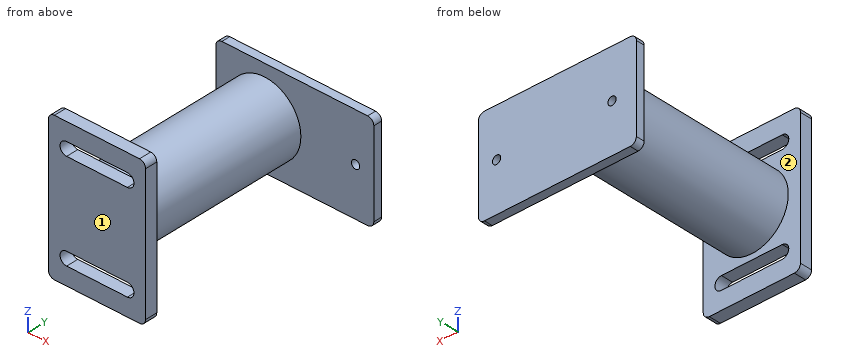
Autodesk Inventor part; units mm, degrees
ref_plane "YZ Plane" through (0, 0, 0) normal (1, 0, 0) x (0, 1, 0)
ref_plane "XZ Plane" through (0, 0, 0) normal (0, 1, 0) x (-1, 0, 0)
ref_plane "XY Plane" through (0, 0, 0) normal (0, 0, 1) x (1, 0, 0)
sketch "Sketch2" plane through (0, 0, 0) normal (0, 1, 0) x (-1, 0, 0)
  line L0 (-25.4, 38.1) -> (25.4, 38.1)
  line L1 (25.4, 38.1) -> (25.4, -38.1)
  line L2 (25.4, -38.1) -> (-25.4, -38.1)
  line L3 (-25.4, -38.1) -> (-25.4, 38.1)
  point P0 (0, 0)
  dimension "d0" = 50.8
  dimension "d1" = 76.2
  dimension "d2" = 25.4
  dimension "d3" = 38.1
extrude "Extrusion1" add sketch "Sketch2" against normal blind 6.35
sketch "Sketch3" plane through (0, 0, 0) normal (0, 1, 0) x (1, 0, 0)
  circle A0 centre (0, 0) radius 19.05
  dimension "d6" = 38.1
extrude "Extrusion2" add sketch "Sketch3" along normal blind 88.9
sketch "Sketch4" plane through (0, 0, 0) normal (0, 1, 0) x (1, 0, 0)
  circle A0 centre (0, 0) radius 19.05
  line L0 (-15.875, 28.829) -> (15.875, 28.829)
  line L1 (15.875, 28.829) -> (15.875, 21.971)
  line L2 (15.875, 21.971) -> (-15.875, 21.971)
  line L3 (-15.875, 21.971) -> (-15.875, 28.829)
  line L4 (-15.875, -21.971) -> (15.875, -21.971)
  line L5 (15.875, -21.971) -> (15.875, -28.829)
  line L6 (15.875, -28.829) -> (-15.875, -28.829)
  line L7 (-15.875, -28.829) -> (-15.875, -21.971)
  line L8 (-15.875, 25.4) -> (15.875, 25.4)
  line L9 (-15.875, -25.4) -> (15.875, -25.4)
  circle A1 centre (-15.875, 25.4) radius 3.429
  circle A2 centre (15.875, 25.4) radius 3.429
  circle A3 centre (15.875, -25.4) radius 3.429
  circle A4 centre (-15.875, -25.4) radius 3.429
  dimension "d10" = 6.858
  dimension "d11" = 6.858
  dimension "d12" = 25.4
  dimension "d14" = 25.4
  dimension "d15" = 31.75
  dimension "d16" = 31.75
  dimension "d17" = 15.875
  dimension "d18" = 15.875
sketch "Sketch5" plane through (0, 88.9, 0) normal (0, 1, 0) x (1, 0, 0)
  circle A0 centre (0, 0) radius 19.05
  line L0 (-25.4, 25.4) -> (57.15, 25.4)
  line L1 (57.15, 25.4) -> (57.15, -25.4)
  line L2 (57.15, -25.4) -> (-25.4, -25.4)
  line L3 (-25.4, -25.4) -> (-25.4, 25.4)
  dimension "d19" = 50.8
  dimension "d20" = 82.55
  dimension "d21" = 25.4
  dimension "d22" = 25.4
extrude "Extrusion3" add sketch "Sketch5" along normal blind 4.445 contours A0 | L0 L1 L2 L3
sketch "Sketch6" plane through (0, 93.345, 0) normal (0, 1, 0) x (1, 0, 0)
  line L0 (-25.4, -25.4) -> (-25.4, 25.4)
  circle A0 centre (-12.7, 0) radius 2.159
  circle A1 centre (47.625, 0) radius 2.159
  point P0 (0, 0)
  dimension "d25" = 4.318
  dimension "d26" = 12.7
  dimension "d27" = 4.318
  dimension "d28" = 60.325
extrude "Extrusion4" cut sketch "Sketch6" against normal blind 10.16
extrude "Extrusion5" cut sketch "Sketch4" against normal blind 6.35 contours A1 L8 L3 | L0 A2 L8 A1 | L3 A1 | A2 L1 | L1 L8 A2 | L8 A1 L3 | L8 A2 L2 A1 | L1 A2 L8 | A4 L9 L7 | L4 A3 L9 A4 | L7 A4 | A3 L5 | L5 L9 A3 | L9 A4 L7 | L9 A3 L6 A4 | L5 A3 L9
fillet "Fillet1" radius 3.175 8 edges at (-25.4, -3.175, 38.1) (25.4, -3.175, 38.1) (25.4, -3.175, -38.1) (-25.4, -3.175, -38.1) (57.15, 91.1225, -25.4) (-25.4, 91.1225, -25.4) (57.15, 91.1225, 25.4) (-25.4, 91.1225, 25.4)
sketch "Sketch7" plane through (0, 93.345, 0) normal (0, 1, 0) x (1, 0, 0)
  arc A0 (-25.4, -22.225) -> (-22.225, -25.4) centre (-22.225, -22.225) ccw
  line L0 (53.975, -25.4) -> (-22.225, -25.4)
  arc A1 (53.975, -25.4) -> (57.15, -22.225) centre (53.975, -22.225) ccw
  line L1 (57.15, 22.225) -> (57.15, -22.225)
  arc A2 (57.15, 22.225) -> (53.975, 25.4) centre (53.975, 22.225) ccw
  line L2 (-22.225, 25.4) -> (53.975, 25.4)
  arc A3 (-22.225, 25.4) -> (-25.4, 22.225) centre (-22.225, 22.225) ccw
  line L3 (-25.4, -22.225) -> (-25.4, 22.225)
  circle A4 centre (47.625, 0) radius 2.159
  circle A5 centre (-12.7, 0) radius 2.159
  point P0 (0, 0)
  dimension "d34" = 60.325
thread "Thread1"
equation "\"d16\" = d15"
equation "\"d17\" = 0.5 * d15"
equation "\"d18\" = d17"
equation "\"d22\" = 0.5 * d19"
properties part number "Lickport_Stand"
CAD build for the part. Positions are in the model's coordinates, mm. Face numbers are marked on the shaded views. A direction names the side the tool comes from. Give positions to 0.01 mm unless a question says otherwise; leave off trailing zeros. Order: outer loops, then holes, each group sorted by start corner. A loop starts at its lowest first (then second) coordinate and runs counter-clockwise, first axis right, second up.
(1) Drill centre lines: L1, parallel to Z at x = 13, y = -1; L2, parallel to X at y = 88.5, z = 0; L3, parallel to Y at x = -14, z = 19 (3 decimals). Where is each one in solid material? Low to high.
(2) Saw through at B-B, the plane z = 20.5. Give the cut face in (x, y) (3 decimals), then the cut area to 3 significant figures.
(3) Saw through at D-D, the plane y = 51. Give the cut face in (x, z).
(4) Flat gauge pins, fed straight in: pin 1 (1 mm diameter, centred on x = -5.5, z = -26, fed in from -Y); pin 2 (8 mm diameter, centred on y = 37.5, z = -19, fed in from -X); pin 3 (1.9 mm diameter, centred on y = -1.5, z = 8.5, fed in from +X); pin 4 (6 mm diameter, centred on x = 17.5, y = 30, fed in from +Z). Where does each tip first touch, or does it go through?
(5) Tool access for the marked faces 1 and 2: list every direction of +Z, -Z, +X, -X, +Y, -Y with a clear straight run to the whole face (end or side of a thin tool).
(6) Saw through at C-C, the plane z = 0. Give the cut face in (x, y) (3 decimals), then the cut area to 3 significant figures.
(7) Saw through at A-A, the plane x = 0. Give the cut face in (y, z) (3 decimals), then the cut area to 3 significant figures.
Results found:
1. L1: z = -38.1 to -28.83, -21.97 to 21.97, 28.83 to 38.1
1. L2: x = -19.05 to -14.86, -10.54 to 19.05
1. L3: y = -6.35 to 0, 88.9 to 93.345
2. outline: (-25.4, -6.35) - (25.4, -6.35) - (25.4, 0) - (-25.4, 0) - close; (-25.4, 88.9) - (57.15, 88.9) - (57.15, 93.345) - (-25.4, 93.345) - close
2. area: 690 mm2
3. outline: circle Ø38.1 at (0, 0)
4. pin 1: passes through
4. pin 2: stops at x = -11.74
4. pin 3: stops at x = 25.4
4. pin 4: stops at z = 12.36
5. face 1: +Z, -Z, +X, -X, -Y
5. face 2: none
6. outline: (-25.4, -6.35) - (25.4, -6.35) - (25.4, 0) - (19.05, 0) - (19.05, 88.9) - (45.466, 88.9) - (45.466, 93.345) - (-10.541, 93.345) - (-10.541, 83.185) - (-14.859, 83.185) - (-14.859, 93.345) - (-25.4, 93.345) - (-25.4, 88.9) - (-19.05, 88.9) - (-19.05, 0) - (-25.4, 0) - close; (49.784, 88.9) - (57.15, 88.9) - (57.15, 93.345) - (49.784, 93.345) - close
6. area: 4,010 mm2
7. outline: (-6.35, -38.1) - (0, -38.1) - (0, -28.829) - (-6.35, -28.829) - close; (-6.35, -21.971) - (0, -21.971) - (0, -19.05) - (88.9, -19.05) - (88.9, -25.4) - (93.345, -25.4) - (93.345, 25.4) - (88.9, 25.4) - (88.9, 19.05) - (0, 19.05) - (0, 21.971) - (-6.35, 21.971) - close; (-6.35, 28.829) - (0, 28.829) - (0, 38.1) - (-6.35, 38.1) - close
7. area: 4,010 mm2
